from build123d import *

# Parameters (mm, degrees)
F1_DEPTH    = 38.1
F2_DEPTH    = 25.4
F3_DEPTH    = 38.1
F4_R        = 3.937
F5_DEPTH    = 6.35
F4_R_2      = 6.35
F6_DEPTH    = 3.175
F6_FACE_R   = 6.35
F6_FACE_R_2 = 3.937
F7_DEPTH    = 12.7
F8_W        = 24.13
F8_H        = 13.208
F9_DEPTH    = 6.35


with BuildPart() as f1:
    # F0 (on Right) → F1 (new body, symmetric)
    with BuildSketch(Plane.YZ):
        Polygon((-38.1, 0), (0, 0), (0, 6.35), (-28.936947, 6.35), (-13.876878, 46.510183), (-11.495628, 52.860183), (5.94569, 99.370366), (0, 101.6), align=None)
    extrude(amount=F1_DEPTH, both=True)

    # F0 (on Right) → F2 (join, symmetric)
    with BuildSketch(Plane.YZ):
        Polygon((-11.495628, 52.860183), (-13.876878, 46.510183), (17.873122, 46.510183), (17.873122, 52.860183), align=None)
    extrude(amount=F2_DEPTH, both=True)

    # F2_face (on face) → F3 (join)
    with BuildSketch(Plane(origin=(25.4, 2.585703, 49.643949), x_dir=(0, 1, 0), z_dir=(1, 0, 0))):
        Polygon((-14.081331, 3.216234), (-16.462581, -3.133766), (15.287419, -3.133766), (15.287419, 3.216234), align=None)
    extrude(amount=F3_DEPTH)

    # F4 (on face) → F5 (cut, through all)
    with BuildSketch(Plane.XY.offset(52.860183)):
        with Locations((50.8, 5.173122)):
            Circle(F4_R)
    extrude(amount=-F5_DEPTH, mode=Mode.SUBTRACT)

    # F4 (on face) → F6 (join)
    with BuildSketch(Plane.XY.offset(52.860183)):
        with Locations((50.8, 5.173122)):
            Circle(F4_R_2)
        with Locations((50.8, 5.173122)):
            Circle(F4_R, mode=Mode.SUBTRACT)
    extrude(amount=F6_DEPTH)

    # F6_face (on face) → F7 (join)
    with BuildSketch(Plane(origin=(50.8, 5.173122, 56.035183), x_dir=(1, 0, 0), z_dir=(0, 0, 1))):
        Circle(F6_FACE_R)
        Circle(F6_FACE_R_2, mode=Mode.SUBTRACT)
    extrude(amount=-F7_DEPTH)

    # F8 (on face) → F9 (cut, through all)
    with BuildSketch(Plane.XY.offset(52.860183)):
        with Locations((-2.062116, 4.919122)):
            Rectangle(F8_W, F8_H)
    extrude(amount=-F9_DEPTH, mode=Mode.SUBTRACT)


solid = f1.part
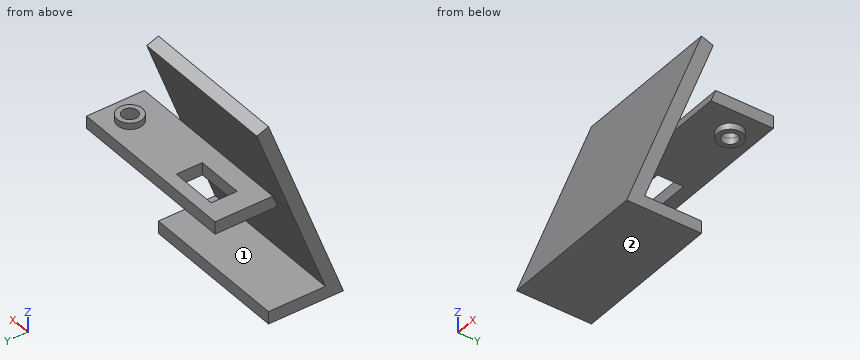
Geometry check sheet. Reference: the model listing, model coordinates, mm. Face numbers are marked on the shaded views. A direction names the side the tool comes from. Give positions to 0.01 mm unless a question says otherwise; leave off trailing zeros. Loops run counter-clockwise (first coordinate to the right, second up) from the corner with the lowest first, then second, coordinate; pieces in that order, holes last. Notation, with made-up numbers: M 23,-5 L 71,-5 A24 cw 71,19 Z; hole C 14,-21 d10. An arc over 180 degrees is marked long. Answer as a JSON object with one key per item and string values. Group by question number.
Item 1: Sectioned sample at C-C on x = -7.5. Record the boundary of the cut face in (y, z).
Item 2: Sectioned sample at D-D on y = -26. Record the boundary of the cut face in (x, z).
Item 3: Sectioned sample at B-B on y = -7. Record the boundary of the cut face in (x, z), plus the area to 3 significant figures.
Item 4: Material ranges on L1, parallel to Y at x = 50.8, z = 44.85; L2, parallel to X at y = 15.5, z = 51; L3, parallel to Y at x = 50.8, z = 49.5, recorded low to high.
Item 5: Access from +Z, -Z, +X, -X, +Y, -Y to the whole of each face (thin tool, end or side, straight path). Record for the marked faces 1 and 2.
Item 6: Gauge pin test, flat ends, axial feed: pin 1 (12.5 mm diameter, centred on x = 50.8, y = 5.17, fed in from -Z); pin 2 (12 mm diameter, centred on x = 39, z = 14.5, fed in from -Y); pin 3 (7 mm diameter, centred on x = -2, z = 3, fed in from +Y); pin 4 (10 mm diameter, centred on y = -25, z = 60.5, fed in from -X). Record the tip position at first contact, or that the pin passes through.
Item 7: Sectioned sample at A-A on x = 50.8. Record the boundary of the cut face in (y, z).
Findings below:
{
 "1": {"outline": "M -38.1,0 L 0,0 L 0,6.35 L -28.94,6.35 L -13.88,46.51 L -1.68,46.51 L -1.68,52.86 L -11.5,52.86 L 5.95,99.37 L 0,101.6 Z; M 11.52,46.51 L 17.87,46.51 L 17.87,52.86 L 11.52,52.86 Z"},
 "2": {"outline": "M -38.1,0 L 38.1,0 L 38.1,6.35 L -38.1,6.35 Z; M -38.1,14.18 L 38.1,14.18 L 38.1,32.27 L -38.1,32.27 Z"},
 "3": {"outline": "M -38.1,0 L 38.1,0 L 38.1,6.35 L -38.1,6.35 Z; M -38.1,64.85 L 38.1,64.85 L 38.1,82.93 L -38.1,82.93 Z; M -25.4,46.51 L 63.5,46.51 L 63.5,52.86 L -25.4,52.86 Z", "area": "2,430 mm2"},
 "4": {"L1": "-1.18 to 1.24, 9.11 to 11.52", "L2": "-25.4 to 63.5", "L3": "-12.76 to 1.24, 9.11 to 17.87"},
 "5": {"face 1": "+X, -X, +Y", "face 2": "-Z, +X, -X, +Y, -Y"},
 "6": {"pin 1": "z = 43.34", "pin 2": "y = -34.89", "pin 3": "y = 0", "pin 4": "through"},
 "7": {"outline": "M -13.88,46.51 L -1.18,46.51 L -1.18,43.34 L 1.24,43.34 L 1.24,56.04 L -1.18,56.04 L -1.18,52.86 L -11.5,52.86 Z; M 9.11,43.34 L 11.52,43.34 L 11.52,46.51 L 17.87,46.51 L 17.87,52.86 L 11.52,52.86 L 11.52,56.04 L 9.11,56.04 Z"}
}
